Geometry check sheet. Reference: the model listing, model coordinates, mm. A direction names the side the tool comes from. Round coordinates to 2 decimals unless told otherwise and drop trailing zeros. Write each loop counter-clockwise with the first axis right and the second up, starting at its lowest first coordinate (ties: lowest second). Pieces come first, ordered by that corner, then holes. Notation, with made-up numbers: (-31.5, -22) -> (0.5, -22) arc R38 cw to (0.5, 17) -> close; hole circle Ø2 at (62.25, -8). An arc over 180 degrees is marked (long way). One line per question, with ' | ' between items.
```python
from build123d import *

# Parameters (mm, degrees)
AUFSATZ_LINEAR_AUSTRAGEN1_DEPTH = 15
SKIZZE2_W                       = 50
SKIZZE2_H                       = 40
AUFSATZ_LINEAR_AUSTRAGEN2_DEPTH = 5


with BuildPart() as part:
    # Skizze1 → Aufsatz-Linear austragen1 (new body)
    with BuildSketch(Plane.XY):
        Polygon((0, 0), (0, 70), (15, 70), (15, 90), (30, 90), (30, 70), (45, 70), (45, 55), (15, 55), (15, 42.5), (35, 42.5), (35, 27.5), (15, 27.5), (15, 0), align=None)
    extrude(amount=AUFSATZ_LINEAR_AUSTRAGEN1_DEPTH)

    # Skizze2 → Aufsatz-Linear austragen2 (add)
    with BuildSketch(Plane.XZ):
        with Locations((22.5, 7.5)):
            Rectangle(SKIZZE2_W, SKIZZE2_H)
    extrude(amount=AUFSATZ_LINEAR_AUSTRAGEN2_DEPTH)


solid = part.part
```
(1) Sectioned sample at A-A on x = 21.5. Record the cut outline in (y, z), then the cut area to 3 significant figures.
Resolved:
outline: (-5, -12.5) -> (0, -12.5) -> (0, 27.5) -> (-5, 27.5) -> close; (27.5, 0) -> (42.5, 0) -> (42.5, 15) -> (27.5, 15) -> close; (55, 0) -> (90, 0) -> (90, 15) -> (55, 15) -> close | area: 950 mm2
(2) Sectioned sample at D-D on y = 26.5. Record the cut outline in (x, z), then the cut area to 3 significant figures.
Resolved:
outline: (0, 0) -> (15, 0) -> (15, 15) -> (0, 15) -> close | area: 225 mm2
(3) Go/stop test with flat-tipped pins: pin 1 (16.5 mm diameter, centred on y = 36, z = 5, fed in from +X); pin 2 (4.5 mm diameter, centred on x = 36, z = 5.5, fed in from +Y); pin 3 (16.5 mm diameter, centred on y = 11.5, z = 6, fed in from +X). Record where each tip stops, or that it passes through.
Resolved:
pin 1: stops at x = 35 | pin 2: stops at y = 70 | pin 3: stops at x = 15
(4) Sectioned sample at B-B on x = 1. Record the cut outline in (y, z), then the cut area to 3 significant figures.
Resolved:
outline: (-5, -12.5) -> (0, -12.5) -> (0, 0) -> (70, 0) -> (70, 15) -> (0, 15) -> (0, 27.5) -> (-5, 27.5) -> close | area: 1,250 mm2
(5) Draft check along Y on faces 4 (the flat face through (22, 90, 7)), 5 (the flat face through (15, 49, 7)), 6 (the flat face through (45, 63, 7)). Enter one of: +Y half, -Y half, draft (parallel to the pull), parting line (faces both ways), or undercut.
Resolved:
face 4: +Y half | face 5: undercut | face 6: draft
(6) Access from +Z, -Z, +X, -X, +Y, -Y to the whole of each face (thin tool, end or side, straight path). Record for faces 1 (the flat face through (15, 80, 7)), 2 (the flat face through (15, 14, 7)), 3 (the flat face through (30, 80, 7)).
Resolved:
face 1: +Z, -Z, -X, +Y | face 2: +Z, -Z, +X | face 3: +Z, -Z, +X, +Y
(7) Material ranges on line 1 (Y direction, x = 31, z = 10.5); line 2 (Z direction, x = 30.5, y = 35.5), recorded low to high.
Resolved:
line 1: y = -5 to 0, 27.5 to 42.5, 55 to 70 | line 2: z = 0 to 15
(8) Sectioned sample at C-C on z = 3.5. Record the cut outline in (x, y), then the cut area to 3 significant figures.
Resolved:
outline: (-2.5, -5) -> (47.5, -5) -> (47.5, 0) -> (15, 0) -> (15, 27.5) -> (35, 27.5) -> (35, 42.5) -> (15, 42.5) -> (15, 55) -> (45, 55) -> (45, 70) -> (30, 70) -> (30, 90) -> (15, 90) -> (15, 70) -> (0, 70) -> (0, 0) -> (-2.5, 0) -> close | area: 2,350 mm2
